Here's how the part is built. I have some questions about the finished solid (model axes, mm). Face numbers are marked on the shaded views. Round coordinates to 2 decimals unless told otherwise and drop trailing zeros. Answer as CSV lines item,"result".
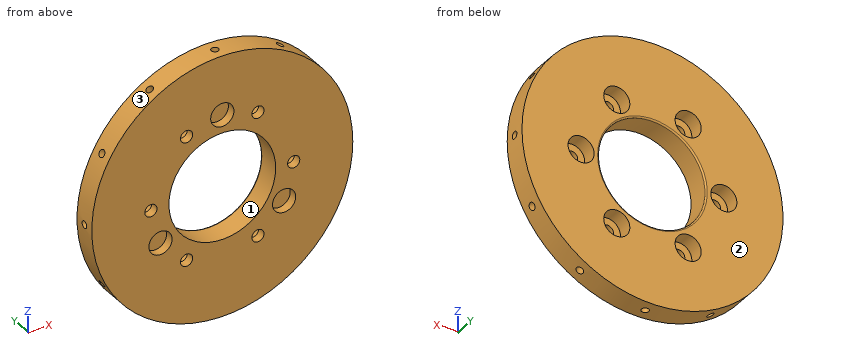
```python
from build123d import *

# Parameters (mm, degrees)
SKETCH_1_R               = 44.975
SKETCH_1_R_2             = 2.1
SKETCH_1_R_3             = 18.4
EXTRUDE_1_DEPTH          = 8
SKETCH_2_R               = 4
CUT_EXTRUDE_1_DEPTH      = 3
SKETCH_4_R               = 4.5
CUT_EXTRUDE_2_DEPTH      = 5.1
SKETCH_5_R               = 1.25
CUT_EXTRUDE_3_DEPTH      = 10
PATTERN_CIRCULAR_1_COUNT = 12
FILLET_1_R               = 0.5


with BuildPart() as part:
    # 草图1 → 凸台-拉伸1 (new body)
    with BuildSketch(Plane(origin=(0, 0, 0), x_dir=(1, 0, 0), z_dir=(0, 1, 0))):
        Circle(SKETCH_1_R)
        with Locations((-24.6, 0)):
            Circle(SKETCH_1_R_2, mode=Mode.SUBTRACT)
        with Locations((-12.3, 21.304224933)):
            Circle(SKETCH_1_R_2, mode=Mode.SUBTRACT)
        with Locations((12.3, 21.304224933)):
            Circle(SKETCH_1_R_2, mode=Mode.SUBTRACT)
        with Locations((24.6, 0)):
            Circle(SKETCH_1_R_2, mode=Mode.SUBTRACT)
        with Locations((12.3, -21.304224933)):
            Circle(SKETCH_1_R_2, mode=Mode.SUBTRACT)
        with Locations((-12.3, -21.304224933)):
            Circle(SKETCH_1_R_2, mode=Mode.SUBTRACT)
        Circle(SKETCH_1_R_3, mode=Mode.SUBTRACT)
    extrude(amount=EXTRUDE_1_DEPTH)

    # 草图2 → 切除-拉伸1 (cut)
    with BuildSketch(Plane.XZ):
        with Locations((-21.304224933, -12.3)):
            Circle(SKETCH_2_R)
        with Locations((0, 24.6)):
            Circle(SKETCH_2_R)
        with Locations((21.304224933, -12.3)):
            Circle(SKETCH_2_R)
    extrude(amount=-CUT_EXTRUDE_1_DEPTH, mode=Mode.SUBTRACT)

    # 草图4 → 切除-拉伸2 (cut)
    with BuildSketch(Plane(origin=(0, 8, 0), x_dir=(1, 0, 0), z_dir=(0, 1, 0))):
        with Locations((-24.6, 0)):
            Circle(SKETCH_4_R)
        with Locations((-12.3, 21.304224933)):
            Circle(SKETCH_4_R)
        with Locations((12.3, 21.304224933)):
            Circle(SKETCH_4_R)
        with Locations((24.6, 0)):
            Circle(SKETCH_4_R)
        with Locations((12.3, -21.304224933)):
            Circle(SKETCH_4_R)
        with Locations((-12.3, -21.304224933)):
            Circle(SKETCH_4_R)
    extrude(amount=-CUT_EXTRUDE_2_DEPTH, mode=Mode.SUBTRACT)

    # 草图5 → 切除-拉伸3 (cut)
    with BuildSketch(Plane(origin=(45, 0, 0), x_dir=(0, 0, -1), z_dir=(1, 0, 0))):
        with Locations((0, 4)):
            Circle(SKETCH_5_R)
    cut_extrude_3 = extrude(amount=-CUT_EXTRUDE_3_DEPTH, mode=Mode.SUBTRACT)

    # 阵列(圆周)1: 切除-拉伸3 ×12 about axis
    pattern_circular_1_axis = Axis((0, 0, 0), (0, 1, 0))
    for i in range(1, PATTERN_CIRCULAR_1_COUNT):
        add(cut_extrude_3.rotate(pattern_circular_1_axis, i * 360 / PATTERN_CIRCULAR_1_COUNT), mode=Mode.SUBTRACT)

    # 圆角1
    fillet_1_edges = [part.edges().sort_by_distance(p)[0] for p in [
        (-18.4, 8, 0),
    ]]
    fillet(fillet_1_edges, radius=FILLET_1_R)


solid = part.part
```
1. We'd pull the mould along Z, two halves only. Please class the marked faces 1, 2 and 3: pulls with the +Z half, pulls with the -Z half, needs draft (parallel to the pull), parting line crosses it, or undercut.
Evaluation:
face 1,"undercut"
face 2,"needs draft"
face 3,"parting line crosses it"
2. If I drill on line 1 (X direction, y = 6, z = 0) (3 decimals); line 2 (X direction, y = 5, z = 0); line 3 (Z direction, x = -12, y = 6.5), over which ranges is the centre line in solid material (lowest first)? Write a range as [from, to].
Evaluation:
line 1,"x = [-44.975, -29.1], [-20.1, -18.4], [18.4, 20.1], [29.1, 44.975]"
line 2,"x = [-35, -29.1], [-20.1, -18.4], [18.4, 20.1], [29.1, 35]"
line 3,"z = [-43.34, -25.79], [-16.81, -13.95], [13.95, 16.81], [25.79, 43.34]"
3. For P1, Ø10, axis at x = -4, z = 19.5, coming from the -Y side; P2, Ø2, axis at y = 2, z = 13.5, coming from the -X side; P3, Ø2, axis at y = 3.5, z = -11, coming from the +X side; P4, Ø1.5, axis at y = 4, z = 0, coming from the -X side, each with a flat end and sliding along its axis, tell me the tip position at first contact or that it passes through.
Evaluation:
P1,"stops at y = 0"
P2,"stops at x = -43.2"
P3,"stops at x = 43.85"
P4,"stops at x = -35"
4. I want a section at A-A, the plane z = 0. Count the separate pieces of the cut face and the enclosed holes in it, and give its area (3 significant figures).
Evaluation:
separate pieces,"4"
enclosed holes,"0"
area,"259 mm²"
